from build123d import *

# Parameters (mm, degrees)
F0_R      = 12.45
F1_DEPTH  = 10
F2_R      = 3
F3_DEPTH  = 10
F4_W      = 3
F4_H      = 6
F5_DEPTH  = 6.5
F6_W      = 3.16
F6_H      = 4.43
F7_DEPTH  = 5.3
F8_W      = 3.16
F8_H      = 0.5056946463
F9_DEPTH  = 4.3
F11_DEPTH = 14.031
F12_W     = 1.2686107075
F12_H     = 0.5
F13_DEPTH = 14.031
F14_DEPTH = 7


with BuildPart() as f1:
    # F0 (on Top) → F1 (new body)
    with BuildSketch(Plane.XY):
        Circle(F0_R)
    extrude(amount=F1_DEPTH)

    # F2 (on face) → F3 (join)
    with BuildSketch(Plane.XY.offset(10)):
        Circle(F2_R)
    extrude(amount=F3_DEPTH)

    # F4 (on face) → F5 (cut)
    with BuildSketch(Plane.XY.offset(10)):
        with Locations((-3, 0)):
            Rectangle(F4_W, F4_H)
    extrude(amount=F5_DEPTH, mode=Mode.SUBTRACT)

    # F6 (on face) → F7 (join)
    with BuildSketch(Plane.XY.offset(20)):
        Rectangle(F6_W, F6_H)
    extrude(amount=F7_DEPTH)

    # F8 (on face) → F9 (cut)
    with BuildSketch(Plane.XY.offset(25.3)):
        with Locations((0, 0.8871526769)):
            Rectangle(F8_W, F8_H)
        with Locations((0, -0.8871526769)):
            Rectangle(F8_W, F8_H)
    extrude(amount=-F9_DEPTH, mode=Mode.SUBTRACT)

    # F10 (on face) → F11 (cut, through all)
    with BuildSketch(Plane(origin=(-1.58, 0, 0), x_dir=(0, -1, 0), z_dir=(-1, 0, 0))):
        Polygon((-2.215, 20), (-1.84, 25.3), (-2.215, 25.3), align=None)
        Polygon((1.84, 25.3), (2.215, 20), (2.215, 25.3), align=None)
    extrude(amount=-F11_DEPTH, mode=Mode.SUBTRACT)

    # F12 (on face) → F13 (cut, through all)
    with BuildSketch(Plane(origin=(-1.58, 0, 0), x_dir=(0, -1, 0), z_dir=(-1, 0, 0))):
        with Locations((0, 25.05)):
            Rectangle(F12_W, F12_H)
    extrude(amount=-F13_DEPTH, mode=Mode.SUBTRACT)

    # F2 (on face) → F14 (cut)
    with BuildSketch(Plane.XY.offset(10)):
        with BuildLine():
            Line((4.9749371855, 0.5), (9.9874921777, 0.5))
            ThreePointArc((9.9874921777, 0.5), (7.0710678119, 7.0710678119), (0.5, 9.9874921777))
            Line((0.5, 9.9874921777), (0.5, 4.9749371855))
            ThreePointArc((0.5, 4.9749371855), (3.5355339059, 3.5355339059), (4.9749371855, 0.5))
        make_face()
        with BuildLine():
            ThreePointArc((0.5, -9.9874921777), (7.0710678119, -7.0710678119), (9.9874921777, -0.5))
            Line((9.9874921777, -0.5), (4.9749371855, -0.5))
            ThreePointArc((4.9749371855, -0.5), (3.5355339059, -3.5355339059), (0.5, -4.9749371855))
            Line((0.5, -4.9749371855), (0.5, -9.9874921777))
        make_face()
        with BuildLine():
            Line((-0.5, -9.9874921777), (-0.5, -4.9749371855))
            ThreePointArc((-0.5, -4.9749371855), (-3.5355339059, -3.5355339059), (-4.9749371855, -0.5))
            Line((-4.9749371855, -0.5), (-9.9874921777, -0.5))
            ThreePointArc((-9.9874921777, -0.5), (-7.0710678119, -7.0710678119), (-0.5, -9.9874921777))
        make_face()
        with BuildLine():
            ThreePointArc((-4.9749371855, 0.5), (-3.5355339059, 3.5355339059), (-0.5, 4.9749371855))
            Line((-0.5, 4.9749371855), (-0.5, 9.9874921777))
            ThreePointArc((-0.5, 9.9874921777), (-7.0710678119, 7.0710678119), (-9.9874921777, 0.5))
            Line((-9.9874921777, 0.5), (-4.9749371855, 0.5))
        make_face()
    extrude(amount=-F14_DEPTH, mode=Mode.SUBTRACT)


solid = f1.part
For this review, take the finished solid that the model builds, in its own axes (mm). A direction names the side the tool comes from. Round coordinates to 2 decimals unless told otherwise and drop trailing zeros. Order: outer loops, then holes, each group sorted by start corner. A loop starts at its lowest first (then second) coordinate and runs counter-clockwise, first axis right, second up. Notation, with made-up numbers: M 31,54 L 85,54 A20 cw 85,59 Z; hole C -14.75,0.25 d5. An arc over 180 degrees is marked long. Use a Markdown table: item, result. Add a question column.
Item 1: Mouldability with a two-part tool opening along X and no side actions: class faces 4 (the flat face through (-1.5, 0, 13)), 5 (the cylindrical face through (-9.18, 8.41, 4.93)), 6 (the flat face through (0.5, 8, 7)), 7 (the flat face through (0, -1.14, 23)) as released by +X, released by -X, zero draft, split by the parting line, or undercut.
Item 2: Add section A-A, the plane z = 23.5. Give the boundary of the cut face in (x, y), then the cut area to 3 significant figures.
Item 3: Add section B-B, the plane y = 0. Give the boundary of the cut face in (x, z), then the cut area to 3 significant figures.
Item 4: Insertion check: pin 1 (12 mm diameter, centred on x = 3, z = 6.5, fed in from -Y); pin 2 (2.5 mm diameter, centred on y = 8.5, z = 8, fed in from -X); pin 3 (1.5 mm diameter, centred on x = -6.5, z = 6, fed in from +Y); pin 4 (1.5 mm diameter, centred on y = 6, z = 7, fed in from +X). Each pin has a flat end and moves straight along its axis. Give the tip position at first contact, or say it passes through.
Item 5: Add section C-C, the plane x = 0. Give the boundary of the cut face in (y, z) (3 decimals).
Item 6: To check wall thickness, follow line 1 along X through (y, z) = (9, 7.75); line 2 along Y through (x, z) = (-1, 3.25); line 3 along Y through (x, z) = (-7, 4.25). State the ranges of each line that lie inside material, in increasing order.
Item 7: Tool access review of faces 1 (the cylindrical face through (-3.57, 3.5, 6.55)), 2 (the flat face through (-0.022, -2.025, 22.687)), 3 (the flat face through (0, 0.634, 23)): name each direction out of +Z, -Z, +X, -X, +Y, -Y from which nothing blocks a thin tool from reaching the whole face with its end or side.
Item 8: Add section D-D, the plane z = 11.25. Give the boundary of the cut face in (x, y), then the cut area to 3 significant figures.
Geometry results:
| question | item | result |
|---|---|---|
| 1 | face 4 | released by -X |
| 1 | face 5 | split by the parting line |
| 1 | face 6 | undercut |
| 1 | face 7 | zero draft |
| 2 | outline | M -1.58,-1.97 L 1.58,-1.97 L 1.58,-1.14 L -1.58,-1.14 Z; M -1.58,-0.63 L 1.58,-0.63 L 1.58,0.63 L -1.58,0.63 Z; M -1.58,1.14 L 1.58,1.14 L 1.58,1.97 L -1.58,1.97 Z |
| 2 | area | 9.24 mm² |
| 3 | outline | M -12.45,0 L 12.45,0 L 12.45,10 L 3,10 L 3,20 L 1.58,20 L 1.58,24.8 L -1.58,24.8 L -1.58,20 L -3,20 L -3,16.5 L -1.5,16.5 L -1.5,10 L -12.45,10 Z |
| 3 | area | 314 mm² |
| 4 | pin 1 | stops at y = -12.45 |
| 4 | pin 2 | stops at x = -10.12 |
| 4 | pin 3 | stops at y = 11.04 |
| 4 | pin 4 | stops at x = 11.29 |
| 5 | outline | M -12.45,0 L 12.45,0 L 12.45,10 L 3,10 L 3,20 L 2.215,20 L 1.84,25.3 L 1.14,25.3 L 1.14,21 L 0.634,21 L 0.634,24.8 L -0.634,24.8 L -0.634,21 L -1.14,21 L -1.14,25.3 L -1.84,25.3 L -2.215,20 L -3,20 L -3,10 L -12.45,10 Z |
| 6 | line 1 | x = -8.6 to -4.36, -0.5 to 0.5, 4.36 to 8.6 |
| 6 | line 2 | y = -12.41 to -9.95, -4.9 to 4.9, 9.95 to 12.41 |
| 6 | line 3 | y = -10.3 to -7.14, -0.5 to 0.5, 7.14 to 10.3 |
| 7 | face 1 | +Z |
| 7 | face 2 | +Z, +X, -X, -Y |
| 7 | face 3 | +Z, +X, -X |
| 8 | outline | M -1.5,-2.6 A3 ccw long -1.5,2.6 Z |
| 8 | area | 22.7 mm² |
